```python
from build123d import *

# Parameters (mm, degrees)
SKETCH1_W           = 44
SKETCH1_H           = 50
BOSS_EXTRUDE1_DEPTH = 10
BOSS_EXTRUDE2_DEPTH = 44
FILLET1_R           = 5
SKETCH3_W           = 94
SKETCH3_H           = 25
BOSS_EXTRUDE3_DEPTH = 30
FILLET2_R           = 10
SKETCH4_R           = 10
CUT_EXTRUDE1_DEPTH  = 3
SKETCH5_R           = 2.5
CUT_EXTRUDE2_DEPTH  = 10
CHAMFER1_SIZE       = 1
FILLET3_R           = 2


with BuildPart() as part:
    # Sketch1 → Boss-Extrude1 (new body)
    with BuildSketch(Plane(origin=(0, 0, 0), x_dir=(1, 0, 0), z_dir=(0, 1, 0))):
        Rectangle(SKETCH1_W, SKETCH1_H)
    extrude(amount=BOSS_EXTRUDE1_DEPTH)

    # Sketch2 → Boss-Extrude2 (add)
    with BuildSketch(Plane(origin=(22, 0, 0), x_dir=(0, 0, -1), z_dir=(1, 0, 0))):
        Polygon((25, 10), (-30.8, 10), (-30.8, -2), (-33, -2), (-33, 10), (-33, 16), (25, 16), align=None)
    extrude(amount=-BOSS_EXTRUDE2_DEPTH)

    # Fillet1
    fillet1_edges = [part.edges().sort_by_distance(p)[0] for p in [
        (22, 5, 25),
        (-22, 5, 25),
        (-22, 8, -25),
        (22, 8, -25),
    ]]
    fillet(fillet1_edges, radius=FILLET1_R)

    # Sketch3 → Boss-Extrude3 (add)
    with BuildSketch(Plane(origin=(0, 16, 0), x_dir=(1, 0, 0), z_dir=(0, 1, 0))):
        with Locations((0, -32.64725537)):
            Rectangle(SKETCH3_W, SKETCH3_H)
    extrude(amount=BOSS_EXTRUDE3_DEPTH)

    # Fillet2
    fillet2_edges = [part.edges().sort_by_distance(p)[0] for p in [
        (47, 31, 45.14725537),
        (47, 31, 20.14725537),
        (-47, 31, 20.14725537),
        (-47, 31, 45.14725537),
    ]]
    fillet(fillet2_edges, radius=FILLET2_R)

    # Sketch4 → Cut-Extrude1 (cut)
    with BuildSketch(Plane.XY.offset(45.14725537)):
        with Locations((0, 31)):
            Circle(SKETCH4_R)
    extrude(amount=-CUT_EXTRUDE1_DEPTH, mode=Mode.SUBTRACT)

    # Sketch5 → Cut-Extrude2 (cut)
    with BuildSketch(Plane.XZ):
        with Locations((0, 5)):
            Circle(SKETCH5_R)
    extrude(amount=-CUT_EXTRUDE2_DEPTH, mode=Mode.SUBTRACT)

    # Chamfer1
    chamfer1_edges = [part.edges().sort_by_distance(p)[0] for p in [
        (-2.5, 0, 5),
    ]]
    chamfer(chamfer1_edges, length=CHAMFER1_SIZE)

    # Fillet3
    fillet3_edges = [part.edges().sort_by_distance(p)[0] for p in [
        (-3.5, 0, 5),
        (0, 0, 25),
        (22, 0, 0),
        (-22, 0, 0),
        (0, 0, -25),
        (20.535533906, 0, 23.535533906),
        (20.535533906, 0, -23.535533906),
        (-20.535533906, 0, -23.535533906),
        (-20.535533906, 0, 23.535533906),
    ]]
    fillet(fillet3_edges, radius=FILLET3_R)


solid = part.part
```
The listing builds one solid part. Answer for the finished solid, in the listing's coordinates (mm). A direction names the side the tool comes from. Coordinates: 2 decimals unless noted, no trailing zeros. Write each loop counter-clockwise with the first axis right and the second up, starting at its lowest first coordinate (ties: lowest second). Pieces come first, ordered by that corner, then holes. Notation, with made-up numbers: (56, -16) -> (71, -16) arc R35 cw to (71, 20) -> close; hole circle Ø7 at (29, 21.25). An arc over 180 degrees is marked (long way). Write each question's results on one line, items separated by ' | '. Start each with the question number.
1) A cutting plane is placed at C-C (z = 5). Determine the outline of the cut face in (x, y).
2) Flat-ended cylindrical pins translate along their axes: pin 1 Ø22 at (x, z) = (-10.5, 0) entering from +Y; pin 2 Ø20 at (y, z) = (9.5, 4) entering from +X; pin 3 Ø6 at (x, y) = (2, 37.5) entering from -Z. Find the tip coordinate at first contact, or state that the pin passes through.
3) A tool of negligible diameter and unlimited length cuts with its end or side. For faces 1 (the flat face through (0, 10, 5)), 2 (the cylindrical face through (21.4, 0.57, -0.28)), 3 (the cylindrical face through (-21.4, 0.57, 0.28)), 4 (the cylindrical face through (21, 6, 23)), 5 (the cylindrical face through (-21, 9, -23)), from which of +Z, -Z, +X, -X, +Y, -Y can it reach the whole face along a straight path? Write none if from no direction.
4) A cutting plane is placed at B-B (x = 0). Determine the outline of the cut face in (y, z).
5) A cutting plane is placed at A-A (y = 31). Determine the outline of the cut face in (x, z), then the cut area to 3 significant figures.
6) A cutting plane is placed at D-D (y = 37.5). Determine the outline of the cut face in (x, z), then the cut area to 3 significant figures.
7) Straight lines are drawn through the part: probe 1 along Z at (x, y) = (0, 3.5); probe 2 along Z at (x, y) = (-8, 3.5); probe 3 along Y at (x, z) = (0, 43.7). For each, find the intervals that lie inside material, in ascending order.
8) For a pull along X with two mould halves and no side action, classify faces 6 (the flat face through (47, 31, 33)), 7 (the flat face through (0, 0, 0)), 8 (the cylindrical face through (-2.17, 21.24, 43.67)) as +X half, -X half, draft (parallel to the pull), parting line (faces both ways), or undercut.
Values follow:
1) outline: (-22, 2) arc R2 ccw to (-20, 0) -> (-4.33, 0) arc R2 ccw to (-2.91, 0.59) -> (-2.5, 1) -> (-2.5, 10) -> (2.5, 10) -> (2.5, 1) -> (2.91, 0.59) arc R2 ccw to (4.33, 0) -> (20, 0) arc R2 ccw to (22, 2) -> (22, 16) -> (-22, 16) -> close
2) pin 1: y = 16 | pin 2: x = 22 | pin 3: z = 20.15
3) face 1: -Y | face 2: -Z, +X, -Y | face 3: -Z, -X, -Y | face 4: +X, -Y | face 5: -Z, -X, +Y, -Y
4) outline: (-2, 30.8) -> (10, 30.8) -> (10, 25) -> (2, 25) arc R2 ccw to (0, 23) -> (0, 9.33) arc R2 ccw to (0.59, 7.91) -> (1, 7.5) -> (10, 7.5) -> (10, 2.5) -> (1, 2.5) -> (0.59, 2.09) arc R2 ccw to (0, 0.67) -> (0, -23) arc R2 ccw to (2, -25) -> (16, -25) -> (16, 20.15) -> (46, 20.15) -> (46, 45.15) -> (41, 45.15) -> (41, 42.15) -> (21, 42.15) -> (21, 45.15) -> (16, 45.15) -> (16, 33) -> (-2, 33) -> close
5) outline: (-47, 30.15) arc R10 ccw to (-37, 20.15) -> (37, 20.15) arc R10 ccw to (47, 30.15) -> (47, 35.15) arc R10 ccw to (37, 45.15) -> (10, 45.15) -> (10, 42.15) -> (-10, 42.15) -> (-10, 45.15) -> (-37, 45.15) arc R10 ccw to (-47, 35.15) -> close | area: 2,200 mm²
6) outline: (-47, 30.15) arc R10 ccw to (-37, 20.15) -> (37, 20.15) arc R10 ccw to (47, 30.15) -> (47, 35.15) arc R10 ccw to (37, 45.15) -> (7.6, 45.15) -> (7.6, 42.15) -> (-7.6, 42.15) -> (-7.6, 45.15) -> (-37, 45.15) arc R10 ccw to (-47, 35.15) -> close | area: 2,220 mm²
7) probe 1: -25 to 2.5, 7.5 to 25, 30.8 to 33 | probe 2: -25 to 25, 30.8 to 33 | probe 3: 16 to 21, 41 to 46
8) face 6: +X half | face 7: draft | face 8: undercut
